Here's the drawing with two shaded views (mm, measured from the low corner). I have some questions. A direction names the side the tool comes from. Coordinates: 2 decimals unless noted, no trailing zeros. Write each loop counter-clockwise with the first axis right and the second up, starting at its lowest first coordinate (ties: lowest second). Pieces come first, ordered by that corner, then holes.
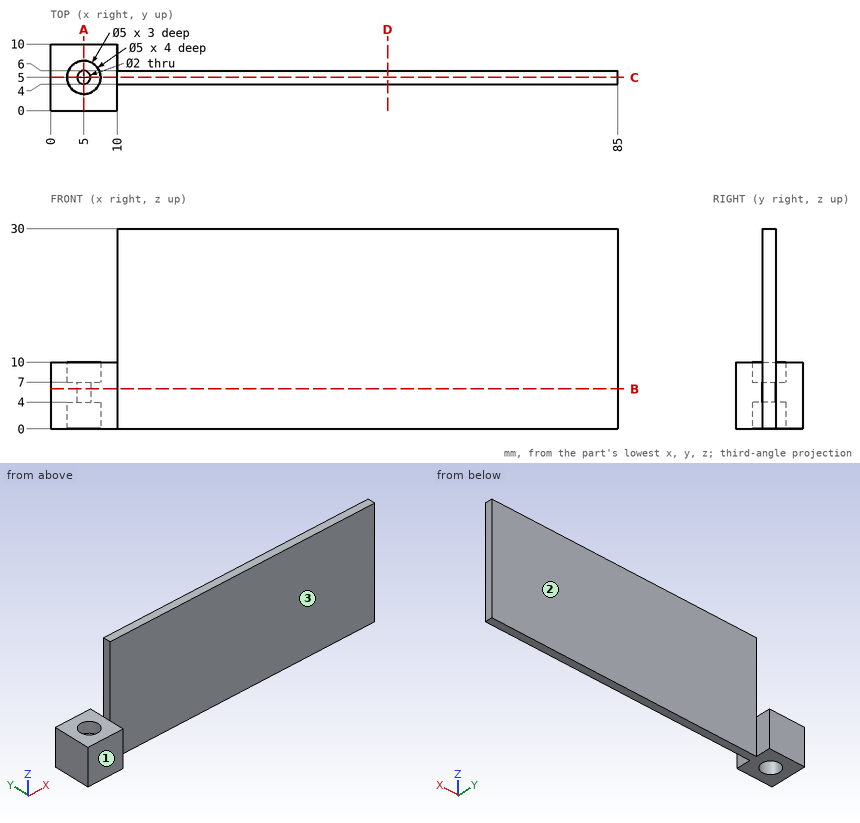
Item 1: Which directions (+Z, -Z, +X, -X, +Y, -Y) give clear straight access to the entire face, cutting with the end or side of a thin tool? Please do the marked faces 1, 2 and 3.
Item 2: I want a section at A-A, the plane x = 5. List the corners of the cut face in (y, z) for me, then the cut area to 3 significant figures.
Item 3: I want a section at D-D, the plane x = 50.5. List the corners of the cut face in (y, z) for me, then the cut area to 3 significant figures.
Item 4: Will these pins go through, and if not, where does the flat tip stop? pin 1 Ø15 at (x, z) = (48, 19.5) entering from -Y; pin 2 Ø3 at (x, y) = (3.5, 5.5) entering from +Z; pin 3 Ø2 at (y, z) = (7.5, 2.5) entering from +X.
Item 5: If I drill on line 1 along Y through (x, z) = (5, 3.1); line 2 along X through (y, z) = (5, 9.45); line 3 along Y through (x, z) = (5, 6.35), over which ranges is the centre line in solid material (lowest first)?
Item 6: I want a section at C-C, the plane y = 5. List the corners of the cut face in (x, z) for me.
Item 7: I want a section at B-B, the plane z = 6. List the corners of the cut face in (x, y) for me, then the cut area to 3 significant figures.
Taken from the geometry:
1. face 1: +Z, -Z, +X, -X, -Y
1. face 2: +Z, -Z, +X, +Y
1. face 3: +Z, -Z, +X, -Y
2. outline: (0, 0) - (2.5, 0) - (2.5, 4) - (4, 4) - (4, 7) - (2.5, 7) - (2.5, 10) - (0, 10) - close; (6, 4) - (7.5, 4) - (7.5, 0) - (10, 0) - (10, 10) - (7.5, 10) - (7.5, 7) - (6, 7) - close
2. area: 59.0 mm2
3. outline: (4, 0) - (6, 0) - (6, 30) - (4, 30) - close
3. area: 60.0 mm2
4. pin 1: stops at y = 4
4. pin 2: stops at z = 10
4. pin 3: stops at x = 10
5. line 1: y = 0 to 2.5, 7.5 to 10
5. line 2: x = 0 to 2.5, 7.5 to 85
5. line 3: y = 0 to 4, 6 to 10
6. outline: (0, 0) - (2.5, 0) - (2.5, 4) - (4, 4) - (4, 7) - (2.5, 7) - (2.5, 10) - (0, 10) - close; (6, 4) - (7.5, 4) - (7.5, 0) - (85, 0) - (85, 30) - (10, 30) - (10, 10) - (7.5, 10) - (7.5, 7) - (6, 7) - close
7. outline: (0, 0) - (10, 0) - (10, 4) - (85, 4) - (85, 6) - (10, 6) - (10, 10) - (0, 10) - close; hole circle Ø2 at (5, 5)
7. area: 247 mm2
